Geometry: final body of the model. Coordinates: model frame, mm. A direction names the side the tool comes from. Round coordinates to 2 decimals unless told otherwise and drop trailing zeros. Order: outer loops, then holes, each group sorted by start corner. A loop starts at its lowest first (then second) coordinate and runs counter-clockwise, first axis right, second up. Notation, with made-up numbers: (-6, -30.5) - (17, -30.5) arc R23 ccw to (17, -8.5) - close; hole circle Ø2 at (78, 30). An arc over 180 degrees is marked (long way). Put each result on its own line as item: value. Start each with the question number.
(1) Pull-direction query (Z, two-part tool) for faces 1 (the face through (0, 9, 2)), 2 (the face through (-0.29, 2.51, 2.32)), 3 (the face through (0, 14.5, 0)); classes: released by +Z, released by -Z, zero draft, split by the parting line, or undercut.
(2) Section C-C (x = -4). Output: boundary loops of the cut face in (y, z), and give its area (3 significant figures).
(3) Pin query (flat end, axial travel): P1, Ø1.3, axis at x = 3.5, z = -0.5, coming from the +Y side; P2, Ø5, axis at y = 11.5, z = 3.5, coming from the -X side; P3, Ø8, axis at x = -5, y = 9, coming from the +Z side. Return the tip coordinate at first contact, or that it passes through.
(4) Material intervals for L1, parallel to Z at x = 0, y = 1.15; L2, parallel to X at y = 2, z = 0.75; L3, parallel to Z at x = 0, y = 0.55, sorted ascending. Write a range as [from, to].
(5) Section B-B (y = 2). Output: boundary loops of the cut face in (x, z), and give its area (3 significant figures).
(6) Section A-A (z = 4). Output: boundary loops of the cut face in (x, y).
(7) Access query for faces 4 (the face through (-4.5, 1.5, 1.4)), 5 (the face through (0, 7, -1)), 6 (the face through (2, 0, 2)). Directions: +Z, -Z, +X, -X, +Y, -Y. A direction counts if a zero-diameter tool reaches every point of the face in a straight line with its end or side. Return the directions, or none.
(8) Section D-D (y = 6.25). Output: boundary loops of the cut face in (x, z), and give its area (3 significant figures).
from build123d import *

# Parameters (mm, degrees)
CBORE_FOR_M2_SHCS1_D           = 2.4
CBORE_FOR_M2_SHCS1_CBORE_D     = 4.4
CBORE_FOR_M2_SHCS1_CBORE_DEPTH = 2
SKETCH8_R                      = 1
CUT_EXTRUDE1_DEPTH             = 14.06
FILLET1_R                      = 1


with BuildPart() as part:
    # Sketch3 → Revolve1 (revolve)
    with BuildSketch(Plane.XY):
        Polygon((0, 0), (0, 14.5), (2, 14.5), (2, 3.5), (8, 3.5), (8, 0), align=None)
    revolve(axis=Axis((0, 0, 0), (0, 1, 0)))

    # CBORE for M2 SHCS1 (through all)
    with Locations(Plane(origin=(0, 3.5, 0), x_dir=(1, 0, 0), z_dir=(0, 1, 0))):
        with Locations((-4.5, 0), (0, 4.5), (4.5, 0), (0, -4.5)):
            CounterBoreHole(CBORE_FOR_M2_SHCS1_D / 2, CBORE_FOR_M2_SHCS1_CBORE_D / 2, CBORE_FOR_M2_SHCS1_CBORE_DEPTH)

    # Sketch8 → Cut-Extrude1 (cut)
    with BuildSketch(Plane.XZ):
        Circle(SKETCH8_R)
    extrude(amount=-CUT_EXTRUDE1_DEPTH, mode=Mode.SUBTRACT)

    # Fillet1
    fillet1_edges = [part.edges().sort_by_distance(p)[0] for p in [
        (-1, 14.06, 0),
        (-1, 0, 0),
    ]]
    fillet(fillet1_edges, radius=FILLET1_R)


solid = part.part
Checks:
1. face 1: split by the parting line
1. face 2: undercut
1. face 3: zero draft
2. outline: (0, -6.93) - (3.5, -6.93) - (3.5, -2.14) - (1.5, -2.14) - (1.5, -1.09) - (0, -1.09) - close; (0, 1.09) - (1.5, 1.09) - (1.5, 2.14) - (3.5, 2.14) - (3.5, 6.93) - (0, 6.93) - close
2. area: 36.7 mm²
3. P1: stops at y = 1.5
3. P2: stops at x = -1.73
3. P3: stops at z = 1.73
4. L1: z = [-8, -5.7], [-3.3, -1], [1, 3.3], [5.7, 8]
4. L2: x = [-7.96, -6.57], [-2.43, -0.66], [0.66, 2.43], [6.57, 7.96]
4. L3: z = [-8, -5.7], [-3.3, -1.11], [1.11, 3.3], [5.7, 8]
5. outline: circle Ø16 at (0, 0); hole circle Ø4.4 at (-4.5, 0); hole circle Ø4.4 at (0, -4.5); hole circle Ø4.4 at (0, 4.5); hole circle Ø2 at (0, 0); hole circle Ø4.4 at (4.5, 0)
5. area: 137 mm²
6. outline: (-6.93, 0) - (-1.09, 0) - (-1.09, 1.5) - (-2.14, 1.5) - (-2.14, 3.5) - (-6.93, 3.5) - close; (1.09, 0) - (6.93, 0) - (6.93, 3.5) - (2.14, 3.5) - (2.14, 1.5) - (1.09, 1.5) - close
7. face 4: +Y
7. face 5: -Y
7. face 6: +Z, -Z, +X, -X, -Y
8. outline: circle Ø4 at (0, 0); hole circle Ø2 at (0, 0)
8. area: 9.42 mm²
